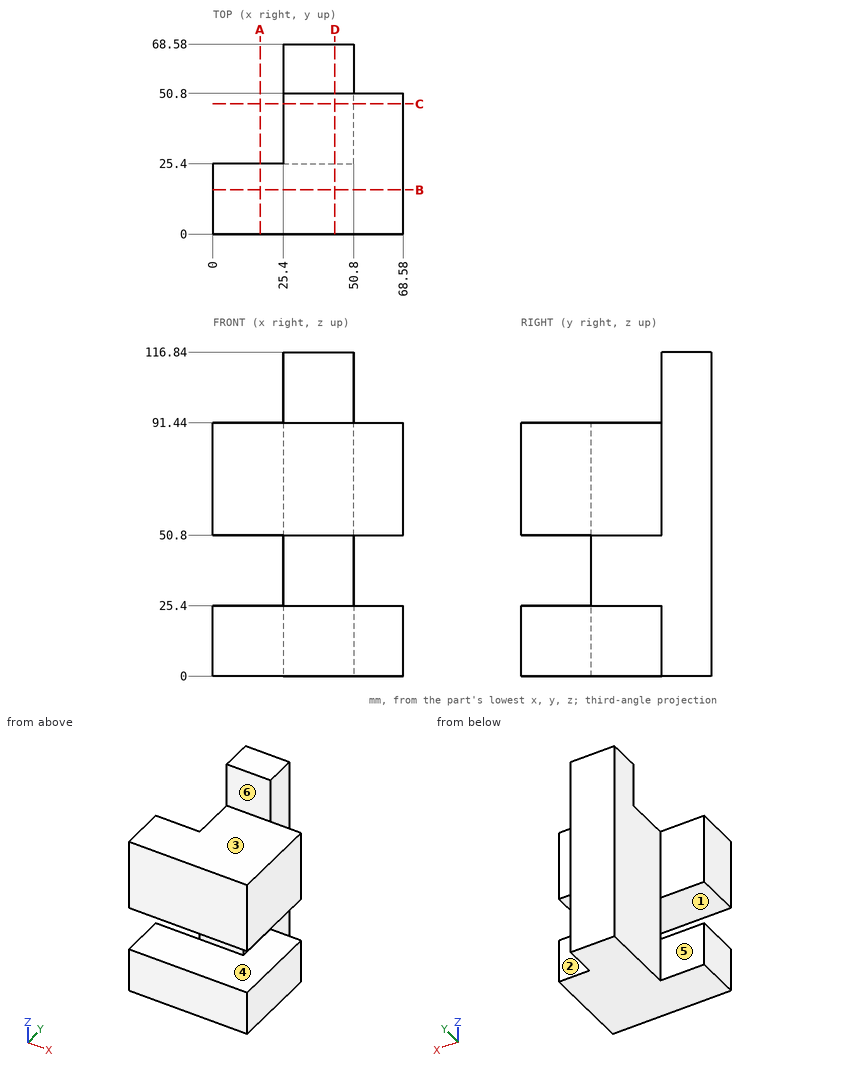
Here's the drawing with two shaded views (mm, measured from the low corner). I have some questions. A direction names the side the tool comes from. Coordinates: 2 decimals unless noted, no trailing zeros. Loops run counter-clockwise (first coordinate to the right, second up) from the corner with the lowest first, then second, coordinate; pieces in that order, holes last. Notation, with made-up numbers: (-11.5, 62.5) -> (22.5, 62.5) arc R13 cw to (22.5, 72.5) -> close; hole circle Ø3 at (15.25, -0.75). An arc over 180 degrees is marked (long way). Answer in a Markdown table with one row per item.
(1) Imagine slicing it at C-C (y = 47). List the corners of the cut face in (x, z) for me.
Results found:
| item | result |
|---|---|
| outline | (25.4, 0) -> (68.58, 0) -> (68.58, 25.4) -> (50.8, 25.4) -> (50.8, 50.8) -> (68.58, 50.8) -> (68.58, 91.44) -> (25.4, 91.44) -> close |
(2) Imagine slicing it at D-D (x = 44). List the corners of the cut face in (y, z) for me, plus the area to 3 significant figures.
Results found:
| item | result |
|---|---|
| outline | (0, 0) -> (68.58, 0) -> (68.58, 116.84) -> (50.8, 116.84) -> (50.8, 91.44) -> (0, 91.44) -> (0, 50.8) -> (25.4, 50.8) -> (25.4, 25.4) -> (0, 25.4) -> close |
| area | 6,080 mm^2 |
(3) Thinking about a two-plate mould opening in Z: for the marked faces 1, 2 and 3, which applies, released by +Z, released by -Z, zero draft, split by the parting line, or undercut?
Results found:
| item | result |
|---|---|
| face 1 | undercut |
| face 2 | zero draft |
| face 3 | released by +Z |
(4) Imagine slicing it at A-A (x = 17). List the corners of the cut face in (y, z) for me, plus the area to 3 significant figures.
Results found:
| item | result |
|---|---|
| outline | (0, 0) -> (25.4, 0) -> (25.4, 25.4) -> (0, 25.4) -> close; (0, 50.8) -> (25.4, 50.8) -> (25.4, 91.44) -> (0, 91.44) -> close |
| area | 1,680 mm^2 |
(5) If I drill on probe 1 along Z at (x, y) = (60.5, 42.5); probe 2 along Y at (x, z) = (56, 80); probe 3 along X at (y, z) = (53.5, 81), over which ranges is the centre line in solid material (lowest first)?
Results found:
| item | result |
|---|---|
| probe 1 | z = 0 to 25.4, 50.8 to 91.44 |
| probe 2 | y = 0 to 50.8 |
| probe 3 | x = 25.4 to 50.8 |
(6) For the marked faces 4, 5 and 6, which set-ups out of +Z, -Z, +X, -X, +Y, -Y let a thin tool reach every point of the face, with its end or its side?
Results found:
| item | result |
|---|---|
| face 4 | +X, -Y |
| face 5 | +Z, -Z, -X, +Y |
| face 6 | +Z, +X, -X, -Y |
(7) Imagine slicing it at B-B (y = 16). List the corners of the cut face in (x, z) for me.
Results found:
| item | result |
|---|---|
| outline | (0, 0) -> (68.58, 0) -> (68.58, 25.4) -> (0, 25.4) -> close; (0, 50.8) -> (68.58, 50.8) -> (68.58, 91.44) -> (0, 91.44) -> close |
(8) Will these pins go through, and if not, where does the flat tip stop? pin 1 Ø12.5 at (x, z) = (11, 12.5) entering from +Y; pin 2 Ø7.5 at (x, z) = (40, 37) entering from -Y; pin 3 Ø12.5 at (x, z) = (37, 107.5) entering from -Y.
Results found:
| item | result |
|---|---|
| pin 1 | stops at y = 25.4 |
| pin 2 | stops at y = 25.4 |
| pin 3 | stops at y = 50.8 |
